from build123d import *

# Parameters (mm, degrees)
F0_W     = 44.45
F0_H     = 44.45
F1_DEPTH = 2.032
F2_R     = 1.5
F3_DEPTH = 6.35
F3_TAPER = 3
F4_R     = 0.254
F5_DEPTH = 25.4
F7_START = 1.016
F6_R     = 4.7625
F7_DEPTH = 1.016


with BuildPart() as f1:
    # F0 (on Top) → F1 (new body)
    with BuildSketch(Plane.XY):
        Rectangle(F0_W, F0_H)
    extrude(amount=F1_DEPTH)

    # F2 (on Top) → F3 (join)
    with BuildSketch(Plane.XY):
        with Locations((-19.304, 9.017)):
            Circle(F2_R)
        with Locations((19.304, 9.017)):
            Circle(F2_R)
    extrude(amount=-F3_DEPTH, taper=F3_TAPER)

    # F4 (on Top) → F5 (cut)
    with BuildSketch(Plane.XY):
        with Locations((-11.049, -6.858)):
            Circle(F4_R)
        with Locations((-11.049, -10.668)):
            Circle(F4_R)
        with Locations((-9.779, -6.858)):
            Circle(F4_R)
        with Locations((-9.779, -10.668)):
            Circle(F4_R)
        with Locations((-8.509, -6.858)):
            Circle(F4_R)
        with Locations((-8.509, -10.668)):
            Circle(F4_R)
    extrude(amount=F5_DEPTH, mode=Mode.SUBTRACT)

    # F6 (on Top) → F7 (cut)
    with BuildSketch(Plane.XY.offset(F7_START)):
        with Locations((-9.779, -8.763)):
            Circle(F6_R)
    extrude(amount=F7_DEPTH, mode=Mode.SUBTRACT)


solid = f1.part
Geometry check sheet. Reference: the model listing, model coordinates, mm. A direction names the side the tool comes from. Coordinates: 2 decimals unless noted, no trailing zeros. Loops run counter-clockwise (first coordinate to the right, second up) from the corner with the lowest first, then second, coordinate; pieces in that order, holes last. Notation, with made-up numbers: (-23, 27.25) - (-5, 27.25) arc R8 cw to (-5, 36.25) - close; hole circle Ø2 at (48, -36). An arc over 180 degrees is marked (long way). Use one line per item in the form item = value. Start each with the question number.
Item 1: Mould release check, pull along X, two halves, no side actions. Record for faces 3 (the face through (0, 22.225, 1)), 4 (the face through (-10, -9, 1.016)), 5 (the face through (-22.225, 0, 1)), 6 (the face through (-18.074, 8.507, -3.219)): +X half, -X half, draft (parallel to the pull), parting line (faces both ways), or undercut.
Item 2: Section check D-D, the plane y = -8. Enter the section's corners in (x, z) (3 decimals), and give its area (3 significant figures).
Item 3: Section check A-A, the plane z = -3.25. Enter the section's corners in (x, y), and give its area (3 significant figures).
Item 4: Section check B-B, the plane y = -16.5. Enter the section's corners in (x, z) (3 decimals).
Item 5: Gauge pin test, flat ends, axial feed: pin 1 (13.5 mm diameter, centred on x = -11, y = 1, fed in from -Z); pin 2 (10.5 mm diameter, centred on x = -9, y = -9, fed in from +Z); pin 3 (8.5 mm diameter, centred on x = -9.779, y = -8.763, fed in from +Z). Record the tip position at first contact, or that the pin passes through.
Item 6: Tool access check on faces 1 (the face through (-5.38, -10.59, 1.52)), 2 (the face through (19, 9, -6.35)). Record the directions out of +Z, -Z, +X, -X, +Y, -Y that give a thin tool (end or side, any length) a straight path to the whole face; none if there is none.
Item 7: Thickness scan on probe 1 along Z at (x, y) = (-17.5, -18.5); probe 2 along X at (y, z) = (-12, 1.75) (3 decimals); probe 3 along X at (y, z) = (9, -5.5). Record the ranges inside material, lowest first.
Computed:
q1.face_3 = draft
q1.face_4 = undercut
q1.face_5 = -X half
q1.face_6 = undercut
q2.outline = (-22.225, 0) - (22.225, 0) - (22.225, 2.032) - (-5.078, 2.032) - (-5.078, 1.016) - (-14.48, 1.016) - (-14.48, 2.032) - (-22.225, 2.032) - close
q2.area = 80.8 mm2
q3.outline = circle Ø2.66 at (-19.3, 9.02); circle Ø2.66 at (19.3, 9.02)
q3.area = 11.1 mm2
q4.outline = (-22.225, 0) - (22.225, 0) - (22.225, 2.032) - (-22.225, 2.032) - close
q5.pin_1 = 0
q5.pin_2 = 2.03
q5.pin_3 = 1.02
q6.face_1 = +Z
q6.face_2 = -Z, +X, -X, +Y, -Y
q7.probe_1 = 0 to 2.03
q7.probe_2 = -22.225 to -13.272, -6.286 to 22.225
q7.probe_3 = -20.52 to -18.09, 18.09 to 20.52
